from build123d import *

# Parameters (mm, degrees)
EXTRUDE_THIN1_DEPTH = 19.05
SKETCH4_R           = 3.175
EXTRUDE3_DEPTH      = 104.450523701
SKETCH9_R           = 3.175
CUT_EXTRUDE3_DEPTH  = 80.552804055
SKETCH8_R           = 4.7625
CUT_EXTRUDE2_DEPTH  = 82.628996839


with BuildPart() as part:
    # Sketch1 → Extrude-Thin1 (new, symmetric)
    with BuildSketch(Plane(origin=(0, 0, 0), x_dir=(1, 0, 0), z_dir=(0, 1, 0))):
        with BuildLine():
            Line((-19.05, -22.225), (-2.032, -22.225))
            ThreePointArc((-2.032, -22.225), (-0.595159021, -21.629840979), (0, -20.193))
            Line((0, -20.193), (0, -5.334))
            ThreePointArc((0, -5.334), (1.562292429, -1.562292429), (5.334, 0))
            Line((5.334, 0), (76.2, 0))
            Line((76.2, 0), (76.2, -3.302))
            Line((76.2, -3.302), (5.334, -3.302))
            ThreePointArc((5.334, -3.302), (3.897159021, -3.897159021), (3.302, -5.334))
            Line((3.302, -5.334), (3.302, -20.193))
            ThreePointArc((3.302, -20.193), (1.739707571, -23.964707571), (-2.032, -25.527))
            Line((-2.032, -25.527), (-19.05, -25.527))
            Line((-19.05, -25.527), (-19.05, -22.225))
        make_face()
    extrude(amount=EXTRUDE_THIN1_DEPTH, both=True)

    # Sketch4 → Extrude3 (cut, through all)
    with BuildSketch(Plane(origin=(-22.225, 0, 25.527), x_dir=(-1, 0, 0), z_dir=(0, 0, -1))):
        with Locations((-11.3792, 10.922)):
            Circle(SKETCH4_R)
        with Locations((-11.3792, -10.922)):
            Circle(SKETCH4_R)
    extrude(amount=EXTRUDE3_DEPTH, mode=Mode.SUBTRACT)

    # Sketch9 → Cut-Extrude3 (cut, through all)
    with BuildSketch(Plane(origin=(3.302, 0, 0), x_dir=(0, 0, -1), z_dir=(1, 0, 0))):
        with Locations((-13.97, 10.922)):
            Circle(SKETCH9_R)
        with Locations((-13.97, -10.922)):
            Circle(SKETCH9_R)
    extrude(amount=-CUT_EXTRUDE3_DEPTH, mode=Mode.SUBTRACT)

    # Sketch8 → Cut-Extrude2 (cut, through all)
    with BuildSketch(Plane.XY.offset(3.302)):
        with Locations((57.7088, 0)):
            Circle(SKETCH8_R)
        with Locations((-12.1412, 0)):
            Circle(SKETCH8_R)
    extrude(amount=-CUT_EXTRUDE2_DEPTH, mode=Mode.SUBTRACT)


solid = part.part
The model under review builds one solid part; all positions refer to its coordinate system, in mm. A direction names the side the tool comes from. Give positions to 0.01 mm unless a question says otherwise; leave off trailing zeros. Loops run counter-clockwise (first coordinate to the right, second up) from the corner with the lowest first, then second, coordinate; pieces in that order, holes last. Notation, with made-up numbers: (26, 60) -> (84, 60) arc R20 cw to (84, 67) -> close; hole circle Ø7 at (75, 7.5). An arc over 180 degrees is marked (long way). Write each question's results on one line, items separated by ' | '.
1) Take a section at B-B, the plane y = 0. Give the boundary of the cut face in (x, z) (3 decimals), plus the area to 3 significant figures.
Conclusion:
outline: (-19.05, 22.225) -> (-2.032, 22.225) arc R2.032 cw to (0, 20.193) -> (0, 5.334) arc R5.334 ccw to (5.334, 0) -> (52.946, 0) -> (52.946, 3.302) -> (5.334, 3.302) arc R2.032 cw to (3.302, 5.334) -> (3.302, 20.193) arc R5.334 ccw to (-2.032, 25.527) -> (-19.05, 25.527) -> close; (62.471, 0) -> (76.2, 0) -> (76.2, 3.302) -> (62.471, 3.302) -> close | area: 346 mm^2
2) Draft analysis for pull direction Y (two halves, no side actions). For faces 4 (the face through (25, -19.05, 2)), 5 (the face through (-19.05, 0, 24)), 6 (the face through (-10.16, 7.82, 23.9)), state which applies: pulls with the +Y half, pulls with the -Y half, needs draft (parallel to the pull), parting line crosses it, or undercut.
Conclusion:
face 4: pulls with the -Y half | face 5: needs draft | face 6: undercut
3) Tool access review of faces 1 (the face through (0, 0, 13)), 2 (the face through (1.67, -9.97, 10.94)), 3 (the face through (3.302, 0, 13)): name each direction out of +Z, -Z, +X, -X, +Y, -Y from which nothing blocks a thin tool from reaching the whole face with its end or side.
Conclusion:
face 1: -Z, -X, +Y, -Y | face 2: +X, -X | face 3: +Z, +X, +Y, -Y
4) Take a section at A-A, the plane z = 13.97. Give the boundary of the cut face in (x, y), plus the area to 3 significant figures.
Conclusion:
outline: (0, -19.05) -> (3.3, -19.05) -> (3.3, -14.1) -> (0, -14.1) -> close; (0, -7.75) -> (3.3, -7.75) -> (3.3, 7.75) -> (0, 7.75) -> close; (0, 14.1) -> (3.3, 14.1) -> (3.3, 19.05) -> (0, 19.05) -> close | area: 83.9 mm^2
5) Insertion check: pin 1 Ø2 at (x, y) = (62, -3) entering from +Z; pin 2 Ø8 at (x, z) = (9, 18.5) entering from -Y; pin 3 Ø1.5 at (y, z) = (-10.5, 18) entering from -X; pin 4 Ø4.5 at (y, z) = (-3.5, 9.5) entering from +X. Each pin has a flat end and moves straight along its axis. Give the tip position at first contact, or say it passes through.
Conclusion:
pin 1: stops at z = 3.3 | pin 2: passes through | pin 3: stops at x = 0 | pin 4: stops at x = 3.3
6) For line 1 along Y through (x, z) = (1.3, 13.97); line 2 along Z through (x, y) = (20, -8), list the stretches that pass through material, from the lowest coordinate up. Write a range as from..to.
Conclusion:
line 1: y = -19.05..-14.1, -7.75..7.75, 14.1..19.05 | line 2: z = 0..3.3
7) Take a section at D-D, the plane x = 15. Give the boundary of the cut face in (y, z).
Conclusion:
outline: (-19.05, 0) -> (19.05, 0) -> (19.05, 3.3) -> (-19.05, 3.3) -> close
8) Take a section at C-C, the plane y = 10. Give the boundary of the cut face in (x, z) (3 decimals), plus the area to 3 significant figures.
Conclusion:
outline: (-19.05, 22.225) -> (-13.884, 22.225) -> (-13.884, 25.527) -> (-19.05, 25.527) -> close; (-7.808, 22.225) -> (-2.032, 22.225) arc R2.032 cw to (0, 20.193) -> (0, 17.008) -> (3.302, 17.008) -> (3.302, 20.193) arc R5.334 ccw to (-2.032, 25.527) -> (-7.808, 25.527) -> close; (0, 5.334) arc R5.334 ccw to (5.334, 0) -> (76.2, 0) -> (76.2, 3.302) -> (5.334, 3.302) arc R2.032 cw to (3.302, 5.334) -> (3.302, 10.932) -> (0, 10.932) -> close | area: 337 mm^2
